```python
from build123d import *

# Parameters (mm, degrees)
SKETCH_1_R          = 16
EXTRUDE_1_DEPTH     = 1.2
SKETCH_2_R          = 7
CUT_EXTRUDE_1_DEPTH = 1.2
SKETCH_3_R          = 0.7
CUT_EXTRUDE_2_DEPTH = 1.2
SKETCH_4_R          = 0.9
EXTRUDE_2_DEPTH     = 6
SKETCH_5_R          = 7
CUT_EXTRUDE_3_DEPTH = 11


with BuildPart() as part:
    # 草图1 → 凸台-拉伸1 (new body)
    with BuildSketch(Plane.XY):
        Circle(SKETCH_1_R)
    extrude(amount=EXTRUDE_1_DEPTH)

    # 草图2 → 切除-拉伸1 (cut)
    with BuildSketch(Plane.XY.offset(1.2)):
        Circle(SKETCH_2_R)
    extrude(amount=-CUT_EXTRUDE_1_DEPTH, mode=Mode.SUBTRACT)

    # 草图3 → 切除-拉伸2 (cut)
    with BuildSketch(Plane.XY.offset(1.2)):
        with Locations((8.660254038, 5)):
            Circle(SKETCH_3_R)
        with Locations((0, -10)):
            Circle(SKETCH_3_R)
        with Locations((-8.660254038, 5)):
            Circle(SKETCH_3_R)
    extrude(amount=-CUT_EXTRUDE_2_DEPTH, mode=Mode.SUBTRACT)

    # 草图4 → 凸台-拉伸2 (add)
    with BuildSketch(Plane(origin=(0, 0, 0), x_dir=(-1, 0, 0), z_dir=(0, 0, -1))):
        with BuildLine():
            Line((1.703894623, 10), (1.703894623, 5.395195442))
            Line((1.703894623, 5.395195442), (-1.703894623, 5.395195442))
            Line((-1.703894623, 5.395195442), (-1.703894623, 10))
            ThreePointArc((-1.703894623, 10), (0, 11.703894623), (1.703894623, 10))
        make_face()
        with Locations((0, 10)):
            Circle(SKETCH_4_R, mode=Mode.SUBTRACT)
        with BuildLine():
            Line((-5.537946003, -1.003403593), (-3.637946003, -4.294300127))
            Line((-3.637946003, -4.294300127), (-7.710254038, -6.645448267))
            ThreePointArc((-7.710254038, -6.645448267), (-10.305702305, -5.95), (-9.610254038, -3.354551733))
            Line((-9.610254038, -3.354551733), (-5.537946003, -1.003403593))
        make_face()
        with Locations((-8.660254038, -5)):
            Circle(SKETCH_4_R, mode=Mode.SUBTRACT)
        with BuildLine():
            Line((3.637946003, -4.294300127), (5.537946003, -1.003403593))
            Line((5.537946003, -1.003403593), (9.610254038, -3.354551733))
            ThreePointArc((9.610254038, -3.354551733), (10.305702305, -5.95), (7.710254038, -6.645448267))
            Line((7.710254038, -6.645448267), (3.637946003, -4.294300127))
        make_face()
        with Locations((8.660254038, -5)):
            Circle(SKETCH_4_R, mode=Mode.SUBTRACT)
    extrude(amount=EXTRUDE_2_DEPTH)

    # 草图5 → 切除-拉伸3 (cut)
    with BuildSketch(Plane.XY.offset(1.2)):
        Circle(SKETCH_5_R)
    extrude(amount=-CUT_EXTRUDE_3_DEPTH, mode=Mode.SUBTRACT)


solid = part.part
```
Geometry check sheet. Reference: the model listing, model coordinates, mm. A direction names the side the tool comes from. Round coordinates to 2 decimals unless told otherwise and drop trailing zeros. Write each loop counter-clockwise with the first axis right and the second up, starting at its lowest first coordinate (ties: lowest second). Pieces come first, ordered by that corner, then holes. Notation, with made-up numbers: (7, 36.5) - (40, 36.5) arc R9 cw to (40, 49.5) - close; hole circle Ø5 at (1.25, 80.5). An arc over 180 degrees is marked (long way). Write each question's results on one line, items separated by ' | '.
(1) Set-up check for faces 1 (the face through (-8.18, -2.53, -2.96)), 2 (the face through (-9, -5, 0)), 3 (the face through (-6.317, -5.841, -2.958)), 4 (the face through (8.22, -2.55, -2.96)): record each of +Z, -Z, +X, -X, +Y, -Y from which the full face is reachable in a straight line by a thin tool's end or side.
Computed:
face 1: -Z, -X, +Y | face 2: -Z | face 3: -Z, -Y | face 4: -Z, +X, +Y
(2) Sectioned sample at A-A, the plane y = 0. Enter the section's corners in (x, z), plus the area to 3 significant figures.
Computed:
outline: (-16, 0) - (-7, 0) - (-7, 1.2) - (-16, 1.2) - close; (7, 0) - (16, 0) - (16, 1.2) - (7, 1.2) - close | area: 21.6 mm^2
(3) Depth check by flat-ended pin: pin 1 Ø1.6 at (y, z) = (9, -4) entering from +X; pin 2 Ø3 at (x, z) = (-3.5, -4.5) entering from +Y; pin 3 Ø4 at (y, z) = (-3.5, -4) entering from +X; pin 4 Ø1.4 at (x, y) = (-8.5, -4.5) entering from -Z. Enter the tip coordinate at first touch or a pass-through.
Computed:
pin 1: stops at x = 1.7 | pin 2: stops at y = -4.9 | pin 3: stops at x = 10.56 | pin 4: stops at z = -6
(4) Draft check along Y on faces 5 (the face through (0, 10, 0)), 6 (the face through (8, -4, -6)), 7 (the face through (6.28, -5.82, -2.96)). Enter one of: pulls with the +Y half, pulls with the -Y half, needs draft (parallel to the pull), parting line crosses it, or undercut.
Computed:
face 5: undercut | face 6: needs draft | face 7: pulls with the -Y half
(5) Sectioned sample at B-B, the plane z = -5.5. Enter the section's corners in (x, y), plus the area to 3 significant figures.
Computed:
outline: (-9.61, -3.35) arc R1.9 ccw to (-7.71, -6.65) - (-4.88, -5.01) arc R7 cw to (-6.78, -1.72) - close; (-1.7, 6.79) arc R7 cw to (1.7, 6.79) - (1.7, 10) arc R1.7 ccw to (-1.7, 10) - close; (4.88, -5.01) - (7.71, -6.65) arc R1.9 ccw to (9.61, -3.35) - (6.78, -1.72) arc R7 cw to start; hole circle Ø1.8 at (-8.66, -5); hole circle Ø1.8 at (0, 10); hole circle Ø1.8 at (8.66, -5) | area: 42.2 mm^2
(6) Sectioned sample at C-C, the plane z = 0.75. Enter the section's corners in (x, y).
Computed:
outline: circle Ø32 at (0, 0); hole circle Ø1.4 at (-8.66, 5); hole circle Ø14 at (0, 0); hole circle Ø1.4 at (0, -10); hole circle Ø1.4 at (8.66, 5)
(7) Sectioned sample at D-D, the plane y = 5. Enter the section's corners in (x, z), plus the area to 3 significant figures.
Computed:
outline: (-15.2, 0) - (-9.36, 0) - (-9.36, 1.2) - (-15.2, 1.2) - close; (-7.96, 0) - (-4.9, 0) - (-4.9, 1.2) - (-7.96, 1.2) - close; (4.9, 0) - (7.96, 0) - (7.96, 1.2) - (4.9, 1.2) - close; (9.36, 0) - (15.2, 0) - (15.2, 1.2) - (9.36, 1.2) - close | area: 21.4 mm^2
(8) Thickness scan on probe 1 along Y at (x, z) = (0, -2.75); probe 2 along Z at (x, y) = (12, -9); probe 3 along Y at (x, z) = (-0.5, -0.75). Record the ranges inside material, lowest first. Write a range as from..to.
Computed:
probe 1: y = 7..9.1, 10.9..11.7 | probe 2: z = 0..1.2 | probe 3: y = 6.98..9.25, 10.75..11.63
